Design review of the part built by this model. Coordinates are the model's own, in mm. A direction names the side the tool comes from. Round coordinates to 2 decimals unless told otherwise and drop trailing zeros. Loops run counter-clockwise (first coordinate to the right, second up) from the corner with the lowest first, then second, coordinate; pieces in that order, holes last. Notation, with made-up numbers: M 65.25,31.25 L 108.25,31.25 A9 ccw 108.25,39.25 Z; hole C 15.5,60.5 d4. An arc over 180 degrees is marked long. One line per item, written item: value. Start each with the question number.
Item 1: Clearance check with flat-ended pins moving along their axes: pin 1 (3 mm diameter, centred on x = 1.65, y = 9.36, fed in from +Z); pin 2 (1.1 mm diameter, centred on x = -2, y = -9.5, fed in from +Z); pin 3 (1.8 mm diameter, centred on x = 21, y = 20, fed in from -Z). State where each tip first meets the part, or that it passes through.
Item 2: For line 1 along Y through (x, z) = (-22, 6.5); line 2 along Y through (x, z) = (-21.5, 7.5); line 3 along X through (y, z) = (19.5, 7.5), list the stretches that pass through material, from the lowest coordinate up.
Item 3: Mouldability with a two-part tool opening along Y and no side actions: class faces 1 (the flat face through (0, 23, 4)), 2 (the flat face through (25, 0, 4)), 3 (the cylindrical face through (-20.13, -20.67, 3.94)) as released by +Y, released by -Y, zero draft, split by the parting line, or undercut.
Item 4: We need section B-B (y = -20). Write out the cut boundary in (x, z), then the cut area to 3 significant figures.
Item 5: We need section A-A (x = -21). Write out the cut boundary in (y, z), then the cut area to 3 significant figures.
Item 6: We need section C-C (x = 12.5). Write out the cut boundary in (y, z), then the cut area to 3 significant figures.
Item 7: For faces 4 (the cylindrical face through (-20.13, 20.67, 3.94)), 5 (the cylindrical face through (-11.332, 2.478, 4.521)), list the 3-axis set-ups (+Z, -Z, +X, -X, +Y, -Y) from which the entire face can be reached by the end or side of a thin tool; tool diameter is ignored.
from build123d import *

# Parameters (mm, degrees)
SKETCH_1_W          = 50
SKETCH_1_H          = 46
EXTRUDE_1_DEPTH     = 8
SKETCH_2_R          = 1.025
CUT_EXTRUDE_1_DEPTH = 5
SKETCH_3_R          = 1.8
CUT_EXTRUDE_2_DEPTH = 2
SKETCH_4_R          = 1.1
CUT_EXTRUDE_3_DEPTH = 24


with BuildPart() as part:
    # 草图1 → 凸台-拉伸1 (new body)
    with BuildSketch(Plane.XY):
        Rectangle(SKETCH_1_W, SKETCH_1_H)
    extrude(amount=EXTRUDE_1_DEPTH)

    # 草图2 → 切除-拉伸1 (cut)
    with BuildSketch(Plane.XY.offset(8)):
        with Locations((-1.649657688, -9.355673654)):
            Circle(SKETCH_2_R)
        with Locations((12.310096913, -2.170602221)):
            Circle(SKETCH_2_R)
        with Locations((1.649657688, 9.355673654)):
            Circle(SKETCH_2_R)
        with Locations((-12.310096913, 2.170602221)):
            Circle(SKETCH_2_R)
    extrude(amount=-CUT_EXTRUDE_1_DEPTH, mode=Mode.SUBTRACT)

    # 草图3 → 切除-拉伸2 (cut)
    with BuildSketch(Plane.XY.offset(8)):
        with Locations((-12.310096913, 2.170602221)):
            Circle(SKETCH_3_R)
        with Locations((1.649657688, 9.355673654)):
            Circle(SKETCH_3_R)
        with Locations((12.310096913, -2.170602221)):
            Circle(SKETCH_3_R)
        with Locations((-1.649657688, -9.355673654)):
            Circle(SKETCH_3_R)
    extrude(amount=-CUT_EXTRUDE_2_DEPTH, mode=Mode.SUBTRACT)

    # 草图4 → 切除-拉伸3 (cut)
    with BuildSketch(Plane(origin=(0, 0, 0), x_dir=(-1, 0, 0), z_dir=(0, 0, -1))):
        with Locations((21, -20)):
            Circle(SKETCH_4_R)
        with Locations((-21, -20)):
            Circle(SKETCH_4_R)
    cut_extrude_3 = extrude(amount=-CUT_EXTRUDE_3_DEPTH, mode=Mode.SUBTRACT)

    # 镜向1: 切除-拉伸3 across plane
    add(cut_extrude_3.mirror(Plane(origin=(0, 0, 0), x_dir=(0, 0, 1), z_dir=(0, -1, 0))), mode=Mode.SUBTRACT)


solid = part.part
A:
1. pin 1: z = 6
1. pin 2: z = 3
1. pin 3: through
2. line 1: -23 to -20.46, -19.54 to 19.54, 20.46 to 23
2. line 2: -23 to -20.98, -19.02 to 19.02, 20.98 to 23
2. line 3: -25 to -21.98, -20.02 to 20.02, 21.98 to 25
3. face 1: released by +Y
3. face 2: zero draft
3. face 3: undercut
4. outline: M -25,0 L -22.1,0 L -22.1,8 L -25,8 Z; M -19.9,0 L 19.9,0 L 19.9,8 L -19.9,8 Z; M 22.1,0 L 25,0 L 25,8 L 22.1,8 Z
4. area: 365 mm2
5. outline: M -23,0 L -21.1,0 L -21.1,8 L -23,8 Z; M -18.9,0 L 18.9,0 L 18.9,8 L -18.9,8 Z; M 21.1,0 L 23,0 L 23,8 L 21.1,8 Z
5. area: 333 mm2
6. outline: M -23,0 L 23,0 L 23,8 L -0.38,8 L -0.38,6 L -1.16,6 L -1.16,3 L -3.18,3 L -3.18,6 L -3.96,6 L -3.96,8 L -23,8 Z
6. area: 355 mm2
7. face 4: +Z, -Z
7. face 5: +Z
